```python
from build123d import *

# Parameters (mm, degrees)
CROQUIS1_R              = 4.826
SALIENTE_EXTRUIR1_DEPTH = 9.652
CROQUIS2_W              = 57.404
CROQUIS2_H              = 1.524
CORTAR_EXTRUIR1_DEPTH   = 91.375559356
CROQUIS4_R              = 3.937
SALIENTE_EXTRUIR2_DEPTH = 7.874
SALIENTE_EXTRUIR3_REACH = 124.386
SALIENTE_EXTRUIR4_START = 14.986
CROQUIS8_R              = 9.525
CROQUIS8_R_2            = 6.35
SALIENTE_EXTRUIR4_DEPTH = 35.052
CROQUIS8_2_R            = 6.35
CORTAR_EXTRUIR2_DEPTH   = 131.731959853
CORTAR_EXTRUIR3_DEPTH   = 131.731959853


with BuildPart() as part:
    # Croquis1 → Saliente-Extruir1 (new body)
    with BuildSketch(Plane(origin=(0, 0, 0), x_dir=(1, 0, 0), z_dir=(0, 1, 0))):
        with BuildLine():
            Line((-34.925, 38.1), (34.925, 38.1))
            ThreePointArc((34.925, 38.1), (43.905256121, 34.380256121), (47.625, 25.4))
            Line((47.625, 25.4), (47.625, -25.4))
            ThreePointArc((47.625, -25.4), (43.905256121, -34.380256121), (34.925, -38.1))
            Line((34.925, -38.1), (-34.925, -38.1))
            ThreePointArc((-34.925, -38.1), (-43.905256121, -34.380256121), (-47.625, -25.4))
            Line((-47.625, -25.4), (-47.625, 25.4))
            ThreePointArc((-47.625, 25.4), (-43.905256121, 34.380256121), (-34.925, 38.1))
        make_face()
        with Locations(Location((-34.925, 25.4, 0), (0, 0, 270))):
            Circle(CROQUIS1_R, mode=Mode.SUBTRACT)
        with Locations(Location((34.925, 25.4, 0), (0, 0, 270))):
            Circle(CROQUIS1_R, mode=Mode.SUBTRACT)
        with Locations(Location((-34.925, -25.4, 0), (0, 0, 270))):
            Circle(CROQUIS1_R, mode=Mode.SUBTRACT)
        with Locations(Location((34.925, -25.4, 0), (0, 0, 270))):
            Circle(CROQUIS1_R, mode=Mode.SUBTRACT)
    extrude(amount=SALIENTE_EXTRUIR1_DEPTH)

    # Croquis2 → Cortar-Extruir1 (cut, through all)
    with BuildSketch(Plane.XY.offset(38.1)):
        with Locations((0, 0.762)):
            Rectangle(CROQUIS2_W, CROQUIS2_H)
    extrude(amount=-CORTAR_EXTRUIR1_DEPTH, mode=Mode.SUBTRACT)



with BuildPart() as body_2:
    # Croquis4 → Saliente-Extruir2 (new body)
    with BuildSketch(Plane(origin=(0, 74.409783942, 42.960508789), x_dir=(0, 0.5000000000000009, -0.866025403784438), z_dir=(0, -0.8660254037844382, -0.500000000000001))):
        with BuildLine():
            Line((58.190432116, -23.876), (13.486432116, -23.876))
            ThreePointArc((13.486432116, -23.876), (7.918673321, -21.569758795), (5.612432116, -16.002))
            Line((5.612432116, -16.002), (5.612432116, 16.002))
            ThreePointArc((5.612432116, 16.002), (7.918673321, 21.569758795), (13.486432116, 23.876))
            Line((13.486432116, 23.876), (58.190432116, 23.876))
            ThreePointArc((58.190432116, 23.876), (63.758190911, 21.569758795), (66.064432116, 16.002))
            Line((66.064432116, 16.002), (66.064432116, -16.002))
            ThreePointArc((66.064432116, -16.002), (63.758190911, -21.569758795), (58.190432116, -23.876))
        make_face()
        with Locations((58.190432116, -16.002)):
            Circle(CROQUIS4_R, mode=Mode.SUBTRACT)
        with Locations((13.486432116, 16.002)):
            Circle(CROQUIS4_R, mode=Mode.SUBTRACT)
        with Locations((13.486432116, -16.002)):
            Circle(CROQUIS4_R, mode=Mode.SUBTRACT)
        with Locations((58.190432116, 16.002)):
            Circle(CROQUIS4_R, mode=Mode.SUBTRACT)
    extrude(amount=-SALIENTE_EXTRUIR2_DEPTH)


with BuildPart() as part_1:
    add(part.part)

    add(body_2.part)  # Saliente-Extruir3 merges body 2
    # Saliente-Extruir3: up to this plane
    saliente_extruir3_end = Plane(origin=(16.002, 103.505, -7.43388368), z_dir=(0, -0.866025403784438, -0.5000000000000009))
    # Croquis5 → Saliente-Extruir3 (add, up to the surface)
    with BuildSketch(Plane(origin=(0, 9.652, 0), x_dir=(1, 0, 0), z_dir=(0, 1, 0)), mode=Mode.PRIVATE) as saliente_extruir3_sk1:
        Polygon((-47.625, 3.937), (47.625, 3.937), (47.625, -3.937), (3.937, -3.937), (3.937, -38.1), (-3.937, -38.1), (-3.937, -3.937), (-47.625, -3.937), align=None)
    saliente_extruir3_tool1 = split(extrude(saliente_extruir3_sk1.sketch, amount=SALIENTE_EXTRUIR3_REACH, mode=Mode.PRIVATE), bisect_by=saliente_extruir3_end, keep=Keep.BOTH, mode=Mode.PRIVATE)
    add(saliente_extruir3_tool1.solids().sort_by_distance((0, 9.652, 5.548554))[0])

    # Croquis6 → Cortar-Recubrir2 section 0
    with BuildSketch(Plane.XY.offset(3.937)):
        with BuildLine():
            Line((23.876, 96.940017246), (47.625, 9.652))
            Line((47.625, 9.652), (47.625, 96.940017246))
            Line((47.625, 96.940017246), (23.876, 96.940017246))
        make_face()
    # Croquis7 → Cortar-Recubrir2 section 1
    with BuildSketch(Plane(origin=(0, 0, -3.937), x_dir=(-1, 0, 0), z_dir=(0, 0, -1))):
        with BuildLine():
            Line((-23.876, 101.486073266), (-47.625, 9.652))
            Line((-47.625, 9.652), (-47.625, 101.486073266))
            Line((-47.625, 101.486073266), (-23.876, 101.486073266))
        make_face()
    cortar_recubrir2 = loft(mode=Mode.SUBTRACT)

    # Simetr_a1: Cortar-Recubrir2 across plane
    add(cortar_recubrir2.mirror(Plane(origin=(0, 0, 0), x_dir=(0, 0, 1), z_dir=(1, 0, 0))), mode=Mode.SUBTRACT)

    # Croquis8 → Saliente-Extruir4 (add)
    with BuildSketch(Plane.XY.offset(3.937).offset(SALIENTE_EXTRUIR4_START)):
        with Locations((12.7, 44.704)):
            Circle(CROQUIS8_R)
        with Locations((12.7, 44.704)):
            Circle(CROQUIS8_R_2, mode=Mode.SUBTRACT)
    extrude(amount=-SALIENTE_EXTRUIR4_DEPTH)

    # Croquis8_2 → Cortar-Extruir2 (cut, through all)
    with BuildSketch(Plane.XY.offset(3.937)):
        with Locations((12.7, 44.704)):
            Circle(CROQUIS8_2_R)
    extrude(amount=-CORTAR_EXTRUIR2_DEPTH, mode=Mode.SUBTRACT)

    # Croquis9 → Cortar-Extruir3 (cut, through all)
    with BuildSketch(Plane.XY.offset(3.937)):
        Polygon((35.501063323, 71.882673058), (25.906181344, 66.845360019), (28.559347202, 61.791710765), (22.462060614, 58.590635306), (28.559347202, 56.691480467), (28.559347202, 46.97675609), (33.208528226, 45.528650525), (30.883937714, 38.065491513), (35.501063323, 38.065491513), (35.501063323, 33.754439669), (44.724683108, 33.754439669), align=None)
    extrude(amount=-CORTAR_EXTRUIR3_DEPTH, mode=Mode.SUBTRACT)


solid = part_1.part
```
Geometry: final body of the model. Coordinates: model frame, mm. A direction names the side the tool comes from. Round coordinates to 2 decimals unless told otherwise and drop trailing zeros. Write each loop counter-clockwise with the first axis right and the second up, starting at its lowest first coordinate (ties: lowest second). Pieces come first, ordered by that corner, then holes. Notation, with made-up numbers: M 65,-38 L 103,-38 A29 cw 103,-3 Z; hole C 38,83.25 d8. An arc over 180 degrees is marked long. Answer in a Markdown table with one row per item. Add a question column.
(1) Cut plane B-B, the plane z = 5.5. Return the cut outline in (x, y) (3 decimals).
(2) Draft query along X for faces 1 (the face through (47.625, 5, 0)), 2 (the face through (-30.14, 4.76, 24.77)), 3 (the face through (22.22, 44.34, 11.53)), 4 (the face through (-21, 43, 3.937)). Return one class per face: pulls with the +X half, pulls with the -X half, needs draft (parallel to the pull), parting line crosses it, or undercut.
(3) Reachability of faces 5 (the face through (0, 1.524, 1)), 6 (the face through (-23.876, 96, 14)), 7 (the face through (0, 27, 38.1)), 8 (the face through (15, 38, -16.129)), 9 (the face through (27.214, 64.354, 0.055)) from +Z, -Z, +X, -X, +Y, -Y: full face, straight path, thin tool, end or side. Return the list, or none.
(4) Contact query for flat-ended pins moving along their axis: pin 1 (4.5 mm diameter, centred on x = 38, z = -1, fed in from +Y); pin 2 (4 mm diameter, centred on y = 50.5, z = -0.5, fed in from +X); pin 3 (5 mm diameter, centred on y = 41, z = 16, fed in from +X). Output: stop coordinate, or through.
(5) Ray query, L1, parallel to X at y = 3.5, z = 25.4 (3 decimals); L2, parallel to X at y = 9.5, z = -23 (3 decimals); L3, parallel to Y at x = -2.5, z = -27. Return the intervals inside material, ascending.
(6) Cut plane A-A, the plane z = -18. Return the cut outline in (x, y) (3 decimals), then the cut area to 3 significant figures.
Established:
| question | item | result |
|---|---|---|
| 1 | outline | M -47.625,0 L -28.702,0 L -28.702,1.524 L 28.702,1.524 L 28.702,0 L 47.625,0 L 47.625,9.652 L 3.937,9.652 L 3.937,40.971 A9.525 ccw long 3.937,48.437 L 3.937,96.038 L 23.876,96.038 L 23.876,105.13 L -23.876,105.13 L -23.876,96.038 L -3.937,96.038 L -3.937,9.652 L -47.625,9.652 Z; hole C 12.7,44.704 d12.7 |
| 2 | face 1 | pulls with the +X half |
| 2 | face 2 | undercut |
| 2 | face 3 | undercut |
| 2 | face 4 | needs draft |
| 3 | face 5 | +Z, -Z, -Y |
| 3 | face 6 | +Z, -X, +Y |
| 3 | face 7 | +Z, +X, -X, -Y |
| 3 | face 8 | -Z, +X, -X, +Y |
| 3 | face 9 | +Z, -Z, +X |
| 4 | pin 1 | y = 33.75 |
| 4 | pin 2 | x = 28.56 |
| 4 | pin 3 | x = 22.15 |
| 5 | L1 | -47.625 to -39.751, -30.099 to 30.099, 39.751 to 47.625 |
| 5 | L2 | -47.625 to -39.112, -30.738 to 30.738, 39.112 to 47.625 |
| 5 | L3 | 1.52 to 9.65 |
| 6 | outline | M -47.625,0 L -28.702,0 L -28.702,1.524 L 28.702,1.524 L 28.702,0 L 47.625,0 L 47.625,9.652 L -47.625,9.652 Z |
| 6 | area | 832 mm² |
